Part model, mm, in its own coordinate system. Face numbers are marked on the shaded views. A direction names the side the tool comes from. Round coordinates to 2 decimals unless told otherwise and drop trailing zeros. Write each loop counter-clockwise with the first axis right and the second up, starting at its lowest first coordinate (ties: lowest second). Pieces come first, ordered by that corner, then holes. Notation, with made-up numbers: M 12.5,-14 L 45.5,-14 A29 cw 45.5,22 Z; hole C 38,25.5 d9. An arc over 180 degrees is marked long. Use a Markdown table: item, result. Add a question column.
1) Two-plate mould, pull along X, no slides. Class the marked faces 1, 2, 3 and 4: released by +X, released by -X, zero draft, split by the parting line, or undercut.
2) Slice it at D-D on x = -11.5. Write the cut outline in (y, z).
3) Slice it at A-A on z = 8.75. Write the cut outline in (x, y), plus the area to 3 significant figures.
4) Drop flat-ended pins along their axis: P1, Ø4.5, axis at x = 2.5, y = 15, coming from the +Z side; P2, Ø1.5, axis at x = 0.5, y = 17, coming from the +Z side; P3, Ø9, axis at x = 6, y = 3.5, coming from the +Z side. Give the stop position or say it passes through.
5) Which spindle directions (+Z, -Z, +X, -X, +Y, -Y) get a long thin tool onto all of the face, cutting with end or side? Do the marked faces 5 and 6. Say none if no direction does.
6) Slice it at B-B on y = 22. Write the cut outline in (x, z).
7) Wall check: probe 1 along Y at (x, z) = (0, 3.7); probe 2 along X at (y, z) = (0, 4.5); probe 3 along X at (y, z) = (0, 9.5). Give the ranges that are in metal, low to high.
8) Slice it at C-C on z = 1.75. Give the number of separate pieces and of enclosed holes in the cut face, plus the area to 3 significant figures.
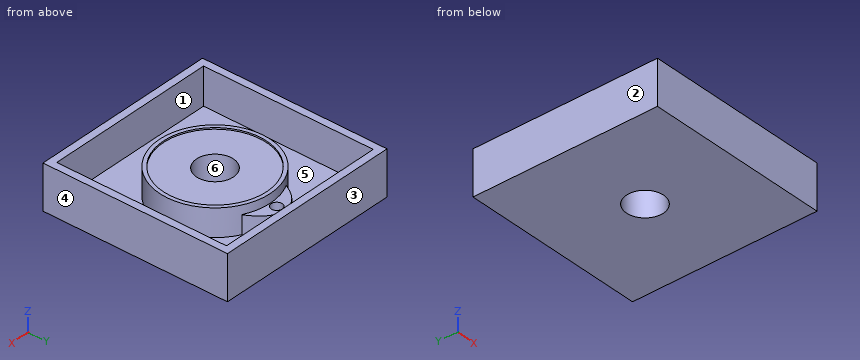
```python
from build123d import *

# Parameters (mm, degrees)
SKETCH_R          = 15
PAD_DEPTH         = 7
SKETCH001_R       = 1.5
PAD001_DEPTH      = 5
SKETCH002_R       = 15
SKETCH002_R_2     = 14
PAD002_DEPTH      = 7.4
SKETCH003_W       = 50
SKETCH003_H       = 50
PAD003_DEPTH      = 2
SKETCH004_W       = 50
SKETCH004_H       = 50
SKETCH004_W_2     = 46
SKETCH004_H_2     = 46
PAD004_DEPTH      = 10
SKETCH005_R       = 5
POCKET_DEPTH      = 2.001
POCKET_DEPTH_BACK = -10.001


with BuildPart() as part:
    # Sketch → Pad (new body)
    with BuildSketch(Plane.XY):
        Circle(SKETCH_R)
    extrude(amount=PAD_DEPTH)

    # Sketch001 → Pad001 (join)
    with BuildSketch(Plane.XY):
        with BuildLine():
            add(Edge.make_bspline(
                [(-6.970964, 13.281779), (-4.960107, 17.400153), (0, 20.361549), (4.960107, 17.400153), (6.970964, 13.281779)],
                knots=[0, 0, 0, 0, 0.5, 1, 1, 1, 1], degree=3))
            Line((6.970964, 13.281779), (-6.970964, 13.281779))
        make_face()
        with Locations((0, 16.734485)):
            Circle(SKETCH001_R, mode=Mode.SUBTRACT)
    extrude(amount=PAD001_DEPTH)

    # Sketch002 → Pad002 (join)
    with BuildSketch(Plane.XY):
        Circle(SKETCH002_R)
        Circle(SKETCH002_R_2, mode=Mode.SUBTRACT)
    extrude(amount=PAD002_DEPTH)

    # Sketch003 → Pad003 (join)
    with BuildSketch(Plane.XY):
        Rectangle(SKETCH003_W, SKETCH003_H)
    extrude(amount=-PAD003_DEPTH)

    # Sketch004 → Pad004 (join)
    with BuildSketch(Plane.XY):
        Rectangle(SKETCH004_W, SKETCH004_H)
        Rectangle(SKETCH004_W_2, SKETCH004_H_2, mode=Mode.SUBTRACT)
    extrude(amount=PAD004_DEPTH)

    # Sketch005 → Pocket (cut, two sides)
    with BuildSketch(Plane.XY) as pocket_sk:
        Circle(SKETCH005_R)
    extrude(amount=-POCKET_DEPTH, mode=Mode.SUBTRACT)
    extrude(pocket_sk.sketch, amount=-POCKET_DEPTH_BACK, mode=Mode.SUBTRACT)


solid = part.part
```
Entries:
| question | item | result |
|---|---|---|
| 1 | face 1 | undercut |
| 1 | face 2 | released by -X |
| 1 | face 3 | zero draft |
| 1 | face 4 | released by +X |
| 2 | outline | M -25,-2 L 25,-2 L 25,10 L 23,10 L 23,0 L 9.63,0 L 9.63,7.4 L 7.98,7.4 L 7.98,7 L -7.98,7 L -7.98,7.4 L -9.63,7.4 L -9.63,0 L -23,0 L -23,10 L -25,10 Z |
| 3 | outline | M -25,-25 L 25,-25 L 25,25 L -25,25 Z; hole M -23,-23 L 23,-23 L 23,23 L -23,23 Z |
| 3 | area | 384 mm^2 |
| 4 | P1 | stops at z = 7.4 |
| 4 | P2 | stops at z = 0 |
| 4 | P3 | stops at z = 7 |
| 5 | face 5 | +Z |
| 5 | face 6 | +Z, -Z |
| 6 | outline | M -25,-2 L 25,-2 L 25,10 L 23,10 L 23,0 L -23,0 L -23,10 L -25,10 Z |
| 7 | probe 1 | y = -25 to -23, -15 to -5, 5 to 15.23, 18.23 to 18.88, 23 to 25 |
| 7 | probe 2 | x = -25 to -23, -15 to -5, 5 to 15, 23 to 25 |
| 7 | probe 3 | x = -25 to -23, 23 to 25 |
| 8 | separate pieces | 2 |
| 8 | enclosed holes | 3 |
| 8 | area | 1,040 mm^2 |
